from build123d import *

# Parameters (mm, degrees)
EXTRUDE_1_DEPTH            = 500
SKETCH_2_W                 = 210
SKETCH_2_H                 = 100
CUT_EXTRUDE_1_DEPTH        = 105
PATTERN_LINEAR_1_COUNT     = 3
PATTERN_LINEAR_1_PITCH     = 270
PATTERN_LINEAR_1_COL_COUNT = 3
PATTERN_LINEAR_1_COL_PITCH = 270


with BuildPart() as part:
    # Sketch 1 → Extrude 1 (new body)
    with BuildSketch(Plane(origin=(0, 0, 0), x_dir=(1, 0, 0), z_dir=(0, 1, 0))):
        Polygon((0, 1032.5), (0, -1032.5), (-265, -654.040778213), (-265, 654.040778213), align=None)
    extrude(amount=EXTRUDE_1_DEPTH)

    # Sketch 2 → Cut-Extrude 1 (cut, symmetric)
    with BuildSketch(Plane.XY):
        with Locations((-105, 450)):
            Rectangle(SKETCH_2_W, SKETCH_2_H)
    cut_extrude_1 = extrude(amount=CUT_EXTRUDE_1_DEPTH, both=True, mode=Mode.SUBTRACT)

    # Pattern Linear 1: Cut-Extrude 1 ×3
    with Locations(*[(0, 0, i * PATTERN_LINEAR_1_PITCH) for i in range(1, PATTERN_LINEAR_1_COUNT)]):
        add(cut_extrude_1, mode=Mode.SUBTRACT)

    # Pattern Linear 1 col: Cut-Extrude 1 ×3
    with Locations(*[(0, 0, -i * PATTERN_LINEAR_1_COL_PITCH) for i in range(1, PATTERN_LINEAR_1_COL_COUNT)]):
        add(cut_extrude_1, mode=Mode.SUBTRACT)


solid = part.part
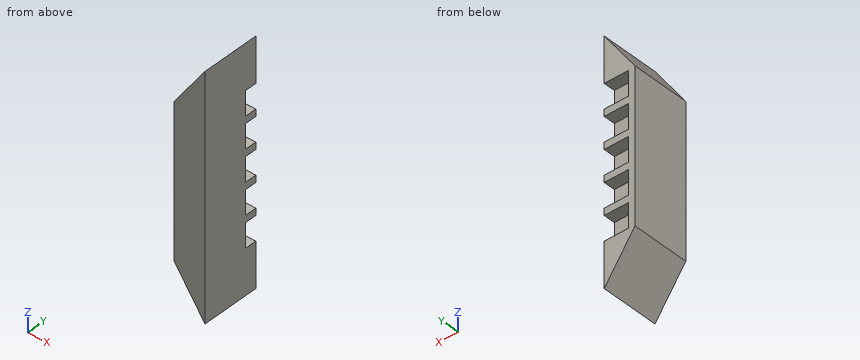
Here's how the part is built. I have some questions about the finished solid (model axes, mm). Coordinates: 2 decimals unless noted, no trailing zeros. Loops run counter-clockwise (first coordinate to the right, second up) from the corner with the lowest first, then second, coordinate; pieces in that order, holes last. Notation, with made-up numbers: (45.25, -36.5) -> (49.25, -36.5) arc R32 cw to (49.25, -9.5) -> close; hole circle Ø10 at (28.25, 71). An arc over 180 degrees is marked (long way). Use one line per item in the form item = value. Start each with the question number.
(1) If we section it at B-B (y = 467.5): Please give me the cut outline in (x, z).
(2) Please list where these lines run through material, in increasing order: line 1 along Z through (x, y) = (-127, 430); line 2 along Z through (x, y) = (-42.5, 477.5); line 3 along Y through (x, z) = (-177.5, 60.5).
(3) Will these pins go through, and if not, where does the flat tip stop? pin 1 (4 mm diameter, centred on x = -106, y = 369.5, fed in from +Z); pin 2 (1 mm diameter, centred on x = -63.5, y = 222, fed in from +Z); pin 3 (1.5 mm diameter, centred on y = 229.5, z = -805, fed in from -X).
(4) If we section it at A-A (z = -576): Please give me the cut outline in (x, y).
(5) If we section it at C-C (x = -161): Please give me the cut outline in (y, z), then the cut area to 3 significant figures.
(6) If we section it at D-D (y = 252.5): Please give me the cut outline in (x, z).
Verdict:
q1.outline = (-265, -654.04) -> (0, -1032.5) -> (0, -645) -> (-210, -645) -> (-210, -435) -> (0, -435) -> (0, -375) -> (-210, -375) -> (-210, -165) -> (0, -165) -> (0, -105) -> (-210, -105) -> (-210, 105) -> (0, 105) -> (0, 165) -> (-210, 165) -> (-210, 375) -> (0, 375) -> (0, 435) -> (-210, 435) -> (-210, 645) -> (0, 645) -> (0, 1032.5) -> (-265, 654.04) -> close
q2.line_1 = -851.13 to -645, -435 to -375, -165 to -105, 105 to 165, 375 to 435, 645 to 851.13
q2.line_2 = -971.8 to -645, -435 to -375, -165 to -105, 105 to 165, 375 to 435, 645 to 971.8
q2.line_3 = 0 to 400
q3.pin_1 = 883.97
q3.pin_2 = 942.53
q3.pin_3 = -159.82
q4.outline = (-265, 0) -> (0, 0) -> (0, 400) -> (-210, 400) -> (-210, 500) -> (-265, 500) -> close
q5.outline = (0, -802.57) -> (500, -802.57) -> (500, -645) -> (400, -645) -> (400, -435) -> (500, -435) -> (500, -375) -> (400, -375) -> (400, -165) -> (500, -165) -> (500, -105) -> (400, -105) -> (400, 105) -> (500, 105) -> (500, 165) -> (400, 165) -> (400, 375) -> (500, 375) -> (500, 435) -> (400, 435) -> (400, 645) -> (500, 645) -> (500, 802.57) -> (0, 802.57) -> close
q5.area = 698,000 mm²
q6.outline = (-265, -654.04) -> (0, -1032.5) -> (0, 1032.5) -> (-265, 654.04) -> close
